Build history of the part. All positions in model axes, mm. A direction names the side the tool comes from. Round coordinates to 2 decimals unless told otherwise and drop trailing zeros. Loops run counter-clockwise (first coordinate to the right, second up) from the corner with the lowest first, then second, coordinate; pieces in that order, holes last. Notation, with made-up numbers: (32.5, 43) - (67.5, 43) arc R20 ccw to (67.5, 62) - close; hole circle Ø5 at (25, 86.25). An arc over 180 degrees is marked (long way). Put each result on its own line as item: value. Start each with the question number.
from build123d import *

# Parameters (mm, degrees)
F1_DEPTH  = 5
F3_DEPTH  = 2.5
F4_SIZE   = 5
F5_R      = 2
F6_R      = 2
F7_D      = 6.6
F7_DEPTH  = 43
F7_TIP    = 1.9828400428
F8_R      = 5
F10_R     = 22.5
F11_DEPTH = 25


with BuildPart() as f1:
    # F0 (on Top) → F1 (new body)
    with BuildSketch(Plane.XY):
        with BuildLine():
            Line((54.1421356237, 17.5), (24.1421356237, 17.5))
            Line((24.1421356237, 17.5), (18.8804864575, 12.2383508337))
            ThreePointArc((18.8804864575, 12.2383508337), (22.5, 0), (18.8804864575, -12.2383508337))
            Line((18.8804864575, -12.2383508337), (24.1421356237, -17.5))
            Line((24.1421356237, -17.5), (54.1421356237, -17.5))
            Line((54.1421356237, -17.5), (54.1421356237, 17.5))
        make_face()
        with BuildLine():
            ThreePointArc((18.8804864575, -12.2383508337), (22.5, 0), (18.8804864575, 12.2383508337))
            Line((18.8804864575, 12.2383508337), (18.8804864575, -12.2383508337))
        make_face()
    extrude(amount=F1_DEPTH)

    # F2 (on Front) → F3 (join, symmetric)
    with BuildSketch(Plane.XZ):
        Polygon((54.1421356237, 20), (18.8804864575, 13), (18.8804864575, 5), (54.1421356237, 5), align=None)
    extrude(amount=F3_DEPTH, both=True)

    # F4
    f4_edges = [f1.edges().sort_by_distance(p)[0] for p in [
        (18.880486, 0, 13),
    ]]
    chamfer(f4_edges, length=F4_SIZE)

    # F5
    f5_edges = [f1.edges().sort_by_distance(p)[0] for p in [
        (23.784784, 0, 13.973581),
    ]]
    fillet(f5_edges, radius=F5_R)

    # F6
    f6_edges = [f1.edges().sort_by_distance(p)[0] for p in [
        (54.142136, 0, 20),
    ]]
    fillet(f6_edges, radius=F6_R)

    # F7
    with Locations(Plane(origin=(0, 0, 0), x_dir=(1, 0, 0), z_dir=(0, 0, -1))):
        with Locations((31.1421356237, -10.5), (46.1421356237, -10.5), (46.1421356237, 10.5), (31.1421356237, 10.5)):
            Hole(F7_D / 2, depth=F7_DEPTH)
            with Locations((0, 0, -(F7_DEPTH + F7_TIP / 2))):  # 118° drill point
                Cone(0, F7_D / 2, F7_TIP, mode=Mode.SUBTRACT)

    # F8
    f8_edges = [f1.edges().sort_by_distance(p)[0] for p in [
        (24.142136, -17.5, 2.5),
        (24.142136, 17.5, 2.5),
        (54.142136, -17.5, 2.5),
        (54.142136, 17.5, 2.5),
    ]]
    fillet(f8_edges, radius=F8_R)

    # F10 (on face) → F11 (cut, symmetric)
    with BuildSketch(Plane(origin=(0, 0, 0), x_dir=(1, 0, 0), z_dir=(0, -0.7071067812, -0.7071067812))):
        Circle(F10_R)
    extrude(amount=F11_DEPTH, both=True, mode=Mode.SUBTRACT)


solid = f1.part
Item 1: Drop flat-ended pins along their axis: pin 1 Ø7.5 at (x, y) = (42, 13.5) entering from +Z; pin 2 Ø4 at (x, z) = (43, 7.5) entering from -Y; pin 3 Ø1 at (x, z) = (39.5, 13) entering from +Y. Give the stop position or say it passes through.
Item 2: Slice it at B-B (x = 24). Give the cut face in (y, z), plus the area to 3 significant figures.
Item 3: Which spindle directions (+Z, -Z, +X, -X, +Y, -Y) get a long thin tool onto all of the face, cutting with end or side? Do faces 5 (the flat face through (37, -2.5, 11)), 6 (the flat face through (38, 10, 5)), 7 (the cylindrical face through (33.76, 12.51, 2.53)). Say none if no direction does.
Item 4: Two-plate mould, pull along Y, no slides. Class faces 1 (the cylindrical face through (52.716, -15.996, 2.535)), 2 (the flat face through (22.305, 0.035, 12.171)), 3 (the cylindrical face through (33.76, -8.49, 2.53)), 4 (the flat face through (21.776, 15.134, 2.465)): pulls with the +Y half, pulls with the -Y half, needs draft (parallel to the pull), parting line crosses it, or undercut.
Item 5: Slice it at C-C (y = 8). Give the number of separate pieces and of enclosed holes in the cut face, plus the area to 3 significant figures.
Item 6: Drill centre lines: probe 1 along X at (y, z) = (9, 1); probe 2 along X at (y, z) = (-10.5, 2.35); probe 3 along Y at (x, z) = (45.5, 1.75). Where is each one in solid material? Low to high. Write a range as [from, to].
Item 7: Slice it at A-A (x = 33.5). Give the cut face in (y, z).
Computed values:
1. pin 1: stops at z = 5
1. pin 2: stops at y = -2.5
1. pin 3: stops at y = 2.5
2. outline: (-16.98, 0) - (16.98, 0) - (16.98, 5) - (2.5, 5) - (2.5, 13.95) - (-2.5, 13.95) - (-2.5, 5) - (-16.98, 5) - close
2. area: 215 mm^2
3. face 5: +Z, +X, -X, -Y
3. face 6: +Z, +X, -X, +Y
3. face 7: +Z, -Z
4. face 1: pulls with the -Y half
4. face 2: needs draft
4. face 3: undercut
4. face 4: pulls with the +Y half
5. separate pieces: 3
5. enclosed holes: 0
5. area: 117 mm^2
6. probe 1: x = [21.78, 28.2], [34.08, 43.2], [49.08, 54.14]
6. probe 2: x = [20.58, 27.84], [34.44, 42.84], [49.44, 54.14]
6. probe 3: y = [-17.5, -13.74], [-7.26, 7.26], [13.74, 17.5]
7. outline: (-17.5, 0) - (-12.81, 0) - (-12.81, 5) - (-17.5, 5) - close; (-8.19, 0) - (8.19, 0) - (8.19, 5) - (2.5, 5) - (2.5, 15.9) - (-2.5, 15.9) - (-2.5, 5) - (-8.19, 5) - close; (12.81, 0) - (17.5, 0) - (17.5, 5) - (12.81, 5) - close
